```python
from build123d import *

# Parameters (mm, degrees)
F1_DEPTH = 3.5
F2_R     = 1.8
F3_DEPTH = 11
F4_R     = 1.8
F5_DEPTH = 7


with BuildPart() as f1:
    # F0 (on Top) → F1 (new body, symmetric)
    with BuildSketch(Plane.XY):
        with BuildLine():
            ThreePointArc((50, 3.5), (45.899495, 13.399495), (36, 17.5))
            Line((36, 17.5), (-36, 17.5))
            ThreePointArc((-36, 17.5), (-45.899495, 13.399495), (-50, 3.5))
            Line((-50, 3.5), (-50, -3.5))
            ThreePointArc((-50, -3.5), (-45.899495, -13.399495), (-36, -17.5))
            Line((-36, -17.5), (36, -17.5))
            ThreePointArc((36, -17.5), (45.899495, -13.399495), (50, -3.5))
            Line((50, -3.5), (50, 3.5))
        make_face()
    extrude(amount=F1_DEPTH, both=True)

    # F2 (on face) → F3 (cut)
    with BuildSketch(Plane.XY.offset(3.5)):
        with Locations((-42.049296, 0)):
            Circle(F2_R)
    extrude(amount=-F3_DEPTH, mode=Mode.SUBTRACT)

    # F4 (on face) → F5 (cut)
    with BuildSketch(Plane.XY.offset(3.5)):
        with Locations((46.846839, 3.143723)):
            Circle(F4_R)
        with Locations((34.45389, -14.343117)):
            Circle(F4_R)
    extrude(amount=-F5_DEPTH, mode=Mode.SUBTRACT)


solid = f1.part
```
The listing builds one solid part. Answer for the finished solid, in the listing's coordinates (mm). Coordinates: 2 decimals unless noted, no trailing zeros. Loops run counter-clockwise (first coordinate to the right, second up) from the corner with the lowest first, then second, coordinate; pieces in that order, holes last. Notation, with made-up numbers: (-7, 7) - (51, 7) arc R10 cw to (51, 23) - close; hole circle Ø2 at (26.5, -5). An arc over 180 degrees is marked (long way). Use a Markdown table: item, result. Add a question column.
1) Given pin 1 (4.5 mm diameter, centred on x = 46.85, y = 3.14, fed in from +Z), flat-ended and moving along its own axis, determine where the tip first touches the part or whether it passes through.
2) The part is cut by section D-D, the plane y = 9.5. Give the vertices of the cut face in (x, z).
3) The part is cut by section B-B, the plane x = -42.5. Give the vertices of the cut face in (y, z).
4) The mould has two halves that part along X. Classify faces 1 (the cylindrical face through (-43.848, 0.079, 0.049)), 2 (the flat face through (-1, 0, 3.5)), 3 (the flat face through (-50, 0, 0)): released by +X, released by -X, zero draft, split by the parting line, or undercut.
5) The part is cut by section C-C, the plane z = 2.5. Give the vertices of the cut face in (x, y).
6) The part is cut by section A-A, the plane y = 0. Give the vertices of the cut face in (x, z).
7) Find the intervals of material crossed by line 1 (X direction, y = 4, z = -0.5); line 2 (X direction, y = -1, z = 2); line 3 (X direction, y = -6, z = 3.25), in increasing order.
Here are the results:
| question | item | result |
|---|---|---|
| 1 | pin 1 | stops at z = 3.5 |
| 2 | outline | (-48.65, -3.5) - (48.65, -3.5) - (48.65, 3.5) - (-48.65, 3.5) - close |
| 3 | outline | (-15.9, -3.5) - (-1.74, -3.5) - (-1.74, 3.5) - (-15.9, 3.5) - close; (1.74, -3.5) - (15.9, -3.5) - (15.9, 3.5) - (1.74, 3.5) - close |
| 4 | face 1 | undercut |
| 4 | face 2 | zero draft |
| 4 | face 3 | released by -X |
| 5 | outline | (-50, -3.5) arc R14 ccw to (-36, -17.5) - (36, -17.5) arc R14 ccw to (50, -3.5) - (50, 3.5) arc R14 ccw to (36, 17.5) - (-36, 17.5) arc R14 ccw to (-50, 3.5) - close; hole circle Ø3.6 at (-42.05, 0); hole circle Ø3.6 at (34.45, -14.34); hole circle Ø3.6 at (46.85, 3.14) |
| 6 | outline | (-50, -3.5) - (-43.85, -3.5) - (-43.85, 3.5) - (-50, 3.5) - close; (-40.25, -3.5) - (50, -3.5) - (50, 3.5) - (-40.25, 3.5) - close |
| 7 | line 1 | x = -49.99 to 45.26, 48.43 to 49.99 |
| 7 | line 2 | x = -50 to -43.55, -40.55 to 50 |
| 7 | line 3 | x = -49.77 to 49.77 |
